Design review of the part built by this model. Coordinates are the model's own, in mm. Face numbers are marked on the shaded views. A direction names the side the tool comes from. Give positions to 0.01 mm unless a question says otherwise; leave off trailing zeros. Order: outer loops, then holes, each group sorted by start corner. A loop starts at its lowest first (then second) coordinate and runs counter-clockwise, first axis right, second up. Notation, with made-up numbers: (80.25, 38.25) -> (123.25, 38.25) arc R23 cw to (123.25, 54.25) -> close; hole circle Ø2 at (-23, 28). An arc over 180 degrees is marked (long way). One line per item, written item: value. Start each with the question number.
1) Consider section A-A (x = 7.5). State the section outline as (y, z) points.
2) Consider section C-C (x = 67.5). State the section outline as (y, z) points, plus the area to 3 significant figures.
3) Wall thickness on line 1 along Y through (x, z) = (4.5, 1); line 2 along Y through (x, z) = (14, 1); line 3 along X through (y, z) = (55, 1.75): over which ranges is each line inside the solid? List them lowest first. Write a range as from..to.
4) For pin 1 (1.4 mm diameter, centred on x = 81, z = 3.5, fed in from +Y); pin 2 (4 mm diameter, centred on y = 52, z = 4, fed in from -X); pin 3 (3 mm diameter, centred on x = 82, z = 3.5, fed in from -Y), all flat-tipped, find the tip position at first contact; note any pin that passes through.
5) Consider section B-B (y = 22). State the section outline as (x, z) points, plus the area to 3 significant figures.
6) Tool access review of the marked faces 1, 2 and 3: name each direction out of +Z, -Z, +X, -X, +Y, -Y from which nothing blocks a thin tool from reaching the whole face with its end or side.
7) Consider section D-D (x = 33). State the section outline as (y, z) points.
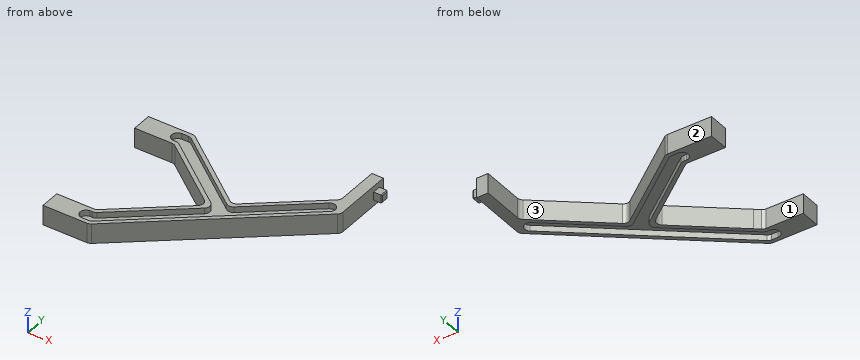
from build123d import *

# Parameters (mm, degrees)
F1_DEPTH = 3.81
F2_DEPTH = 1.5875
F0_W     = 3.175
F0_H     = 3.175
F3_DEPTH = 1.5875
F4_R     = 2.28599
F5_SIZE  = 0.3302


# Not quite as in the source:
# - a fillet or chamfer is up to 0.001 mm smaller than in the source, because OpenCascade refuses the exact size


with BuildPart() as f1:
    # F0 (on Top) → F1 (new body, symmetric)
    with BuildSketch(Plane.XY):
        Polygon((0, 17.9811139863), (0, 10.3611139863), (17.78, 10.3611139863), (80.1876843047, 60.4647179591), (80.1876843047, 78.6070511723), (80.1876843047, 81.7820511723), (80.1876843047, 84.0045511723), (75.7426843047, 84.0045511723), (75.7426843047, 66.6679901496), (48.789068088, 45.0284544481), (17.78, 68.9081139863), (0, 68.9081139863), (0, 61.2881139863), (15.1859866786, 61.2881139863), (15.5029622538, 61.0440154278), (42.6746095935, 40.1195011625), (17.78, 20.1330255541), (15.0996375684, 17.9811139863), align=None)
        Polygon((11.684, 67.3841139863), (17.2611973357, 67.3841139863), (48.8086871908, 43.0898232038), (75.5083847301, 64.5255019445), (78.3706676759, 60.9603202747), (17.2439275137, 11.8851139863), (11.684, 11.8851139863), (11.684, 16.4571139863), (15.6357100547, 16.4571139863), (45.1400120941, 40.1444512324), (15.7047893428, 62.8121139863), (11.684, 62.8121139863), align=None, mode=Mode.SUBTRACT)
    extrude(amount=F1_DEPTH, both=True)

    # F0 (on Top) → F2 (join, symmetric)
    with BuildSketch(Plane.XY):
        Polygon((48.8086871908, 43.0898232038), (17.2611973357, 67.3841139863), (11.684, 67.3841139863), (11.684, 62.8121139863), (15.7047893428, 62.8121139863), (45.1400120941, 40.1444512324), (15.6357100547, 16.4571139863), (11.684, 16.4571139863), (11.684, 11.8851139863), (17.2439275137, 11.8851139863), (78.3706676759, 60.9603202747), (75.5083847301, 64.5255019445), align=None)
    extrude(amount=F2_DEPTH, both=True)

    # F0 (on Top) → F3 (join, symmetric)
    with BuildSketch(Plane.XY):
        with Locations((81.7751843047, 80.1945511723)):
            Rectangle(F0_W, F0_H)
    extrude(amount=F3_DEPTH, both=True)

    # F4 (radius 2.286 in the source; OpenCascade refuses exactly that, so slightly less here)
    f4_edges = [f1.edges().sort_by_distance(p)[0] for p in [
        (15.185987, 61.288114, 0),
        (11.684, 62.812114, 2.69875),
        (15.704789, 62.812114, 2.69875),
        (11.684, 67.384114, 2.69875),
        (17.261197, 67.384114, 2.69875),
        (17.78, 68.908114, 0),
        (15.704789, 62.812114, -2.69875),
        (11.684, 62.812114, -2.69875),
        (11.684, 67.384114, -2.69875),
        (17.261197, 67.384114, -2.69875),
        (48.808687, 43.089823, 2.69875),
        (45.140012, 40.144451, 2.69875),
        (42.67461, 40.119501, 0),
        (48.789068, 45.028454, 0),
        (48.808687, 43.089823, -2.69875),
        (45.140012, 40.144451, -2.69875),
        (75.508385, 64.525502, -2.69875),
        (78.370668, 60.96032, -2.69875),
        (80.187684, 60.464718, 0),
        (75.742684, 66.66799, 0),
        (78.370668, 60.96032, 2.69875),
        (75.508385, 64.525502, 2.69875),
        (15.63571, 16.457114, 2.69875),
        (11.684, 16.457114, 2.69875),
        (11.684, 11.885114, 2.69875),
        (17.243928, 11.885114, 2.69875),
        (11.684, 16.457114, -2.69875),
        (15.63571, 16.457114, -2.69875),
        (17.243928, 11.885114, -2.69875),
        (11.684, 11.885114, -2.69875),
        (17.78, 10.361114, 0),
        (15.099638, 17.981114, 0),
    ]]
    fillet(f4_edges, radius=F4_R)

    # F5
    f5_edges = [f1.edges().sort_by_distance(p)[0] for p in [
        (83.362684, 78.607051, 0),
        (83.362684, 80.194551, -1.5875),
        (83.362684, 81.782051, 0),
        (83.362684, 80.194551, 1.5875),
    ]]
    chamfer(f5_edges, length=F5_SIZE)


with BuildPart() as f1_1:
    # F6: moved
    add(f1.part.moved(Location((0, 0, 3.81))))


solid = f1_1.part
Checked values:
1. outline: (10.36, 0) -> (17.98, 0) -> (17.98, 7.62) -> (10.36, 7.62) -> close; (61.29, 0) -> (68.91, 0) -> (68.91, 7.62) -> (61.29, 7.62) -> close
2. outline: (50.28, 0) -> (52.23, 0) -> (52.23, 2.22) -> (58.1, 2.22) -> (58.1, 0) -> (60.05, 0) -> (60.05, 7.62) -> (58.1, 7.62) -> (58.1, 5.4) -> (52.23, 5.4) -> (52.23, 7.62) -> (50.28, 7.62) -> close
2. area: 48.4 mm^2
3. line 1: y = 10.36..17.98, 61.29..68.91
3. line 2: y = 10.36..11.89, 16.46..17.98, 61.29..62.81, 67.38..68.91
3. line 3: x = 23.35..25.85, 33.34..35.84, 61.21..63.64, 70.95..73.38
4. pin 1: stops at y = 81.78
4. pin 2: stops at x = 24.65
4. pin 3: stops at y = 78.61
5. outline: (20.11, 0) -> (22.54, 0) -> (22.54, 2.22) -> (29.84, 2.22) -> (29.84, 0) -> (32.28, 0) -> (32.28, 7.62) -> (29.84, 7.62) -> (29.84, 5.4) -> (22.54, 5.4) -> (22.54, 7.62) -> (20.11, 7.62) -> close
5. area: 60.3 mm^2
6. face 1: +Z, -Z, -X
6. face 2: +Z, -Z, -X, +Y
6. face 3: +Z, -Z, +Y
7. outline: (22.58, 0) -> (24.53, 0) -> (24.53, 2.22) -> (30.4, 2.22) -> (30.4, 0) -> (32.35, 0) -> (32.35, 7.62) -> (30.4, 7.62) -> (30.4, 5.4) -> (24.53, 5.4) -> (24.53, 7.62) -> (22.58, 7.62) -> close; (47.57, 0) -> (49.49, 0) -> (49.49, 2.22) -> (55.26, 2.22) -> (55.26, 0) -> (57.19, 0) -> (57.19, 7.62) -> (55.26, 7.62) -> (55.26, 5.4) -> (49.49, 5.4) -> (49.49, 7.62) -> (47.57, 7.62) -> close
